Work out the finished part from the listing and answer in its coordinate system (mm). A direction names the side the tool comes from. Round coordinates to 2 decimals unless told otherwise and drop trailing zeros. Answer as CSV lines item,"result". Start each with the question number.
Q1. Each of these flat-tipped pins is pushed along its axis until it touches: pin 1 Ø3 at (x, y) = (-11, 4) entering from +Z; pin 2 Ø0.9 at (y, z) = (4, 151) entering from -X; pin 3 Ø0.5 at (y, z) = (4.5, 140.5) entering from +X; pin 4 Ø3 at (x, y) = (0, 0) entering from -Z. Where does it stop, or does it pass through?
Q2. The mould has two halves that part along Y. Classify faces 4 (the face through (-7, -3.5, 213)), 5 (the face through (-3.5, 2, 213)), 6 (the face through (1.3, 1.9, 0)): +Y half, -Y half, draft (parallel to the pull), parting line (faces both ways), or undercut.
Q3. Straight lines are drawn through the part: L1, parallel to X at y = -0.5, z = 326.5; L2, parallel to Y at x = -11.5, z = 175; L3, parallel to Y at x = 7, z = 354. For each, find the intervals that lie inside material, in ascending order. Write a range as [from, to].
Q4. For faces 1 (the face through (1.3, 1.9, 431.8)), 2 (the face through (11, 2.5, 213)), 3 (the face through (11, 0.5, 213)), determine the directions among +Z, -Z, +X, -X, +Y, -Y from which every point of the face is accessible in a straight line to the end or side of a thin tool.
```python
from build123d import *

# Parameters (mm, degrees)
PAD_DEPTH       = 431.8
FILLET_R        = 1
CHAMFER_SIZE    = 0.5
CHAMFER001_SIZE = 2
FILLET001_R     = 3.5
FILLET002_R     = 1
CHAMFER002_SIZE = 2
FILLET003_R     = 1


with BuildPart() as part:
    # Sketch → Pad (new body)
    with BuildSketch(Plane.XY):
        with BuildLine():
            Line((-13.5, -3.5), (3.75, -3.5))
            Line((3.75, -3.5), (3.75, 0.2))
            Line((3.75, 0.2), (5.75, 0.2))
            Line((5.75, 0.2), (5.75, -3.5))
            Line((5.75, -3.5), (8, -3.5))
            Line((8, -3.5), (8, -1.5))
            Line((8, -1.5), (6.75, -1.5))
            Line((6.75, -1.5), (6.75, 0.5))
            Line((6.75, 0.5), (15.75, 0.5))
            Line((15.75, 0.5), (15.75, -1.5))
            Line((15.75, -1.5), (14.5, -1.5))
            Line((14.5, -1.5), (14.5, -3.5))
            Line((14.5, -3.5), (19.3, -3.5))
            Line((19.3, -3.5), (19.3, -2.5))
            Line((19.3, -2.5), (17.3, -2.5))
            Line((17.3, -2.5), (17.3, -0.7))
            Line((17.3, -0.7), (19.3, -0.7))
            Line((19.3, -0.7), (19.3, 2.5))
            Line((19.3, 2.5), (4.5, 2.5))
            Line((4.5, 2.5), (4.5, 5.25))
            Line((4.5, 5.25), (1, 5.25))
            Line((1, 5.25), (1, 1.732051))
            ThreePointArc((-1, 1.732051), (0, -2), (1, 1.732051))
            Line((-1, 1.732051), (-1, 6.5))
            Line((-1, 6.5), (-16.5, 6.5))
            Line((-16.5, 6.5), (-16.5, 5))
            Line((-16.5, 5), (-13.5, 5))
            Line((-13.5, 5), (-13.5, 3.25))
            Line((-13.5, 3.25), (-11.3, 3.25))
            Line((-11.3, 3.25), (-11.3, 4.15))
            Line((-11.3, 4.15), (-9.5, 4.15))
            Line((-9.5, 4.15), (-9.5, 3.25))
            Line((-9.5, 3.25), (-8.5, 3.25))
            Line((-8.5, 3.25), (-8.5, 5))
            Line((-8.5, 5), (-3.5, 5))
            Line((-3.5, 5), (-3.5, -2))
            Line((-3.5, -2), (-8.5, -2))
            Line((-8.5, -2), (-8.5, -0.25))
            Line((-8.5, -0.25), (-9.5, -0.25))
            Line((-9.5, -0.25), (-9.5, -1.15))
            Line((-9.5, -1.15), (-11.3, -1.15))
            Line((-11.3, -1.15), (-11.3, -0.25))
            Line((-11.3, -0.25), (-13.5, -0.25))
            Line((-13.5, -0.25), (-13.5, -0.45))
            Line((-13.5, -0.45), (-13.3, -0.45))
            Line((-13.3, -0.45), (-13.3, -3.3))
            Line((-13.3, -3.3), (-13.5, -3.3))
            Line((-13.5, -3.3), (-13.5, -3.5))
        make_face()
    extrude(amount=PAD_DEPTH)

    # Fillet
    fillet_edges = [part.edges().sort_by_distance(p)[0] for p in [
        (-1, 6.5, 215.9),
    ]]
    fillet(fillet_edges, radius=FILLET_R)

    # Chamfer
    chamfer_edges = [part.edges().sort_by_distance(p)[0] for p in [
        (4.5, 5.25, 215.9),
    ]]
    chamfer(chamfer_edges, length=CHAMFER_SIZE)

    # Chamfer001
    chamfer001_edges = [part.edges().sort_by_distance(p)[0] for p in [
        (1, 5.25, 215.9),
    ]]
    chamfer(chamfer001_edges, length=CHAMFER001_SIZE)

    # Fillet001
    fillet001_edges = [part.edges().sort_by_distance(p)[0] for p in [
        (3.75, -3.5, 215.9),
    ]]
    fillet(fillet001_edges, radius=FILLET001_R)

    # Fillet002
    fillet002_edges = [part.edges().sort_by_distance(p)[0] for p in [
        (8, -3.5, 215.9),
        (14.5, -3.5, 215.9),
    ]]
    fillet(fillet002_edges, radius=FILLET002_R)

    # Chamfer002
    chamfer002_edges = [part.edges().sort_by_distance(p)[0] for p in [
        (19.3, 2.5, 215.9),
    ]]
    chamfer(chamfer002_edges, length=CHAMFER002_SIZE)

    # Fillet003
    fillet003_edges = [part.edges().sort_by_distance(p)[0] for p in [
        (-16.5, 5, 215.9),
    ]]
    fillet(fillet003_edges, radius=FILLET003_R)


solid = part.part
```
Findings:
1,pin 1,"stops at z = 431.8"
1,pin 2,"stops at x = -13.5"
1,pin 3,"stops at x = 4.5"
1,pin 4,"passes through"
2,face 4,"-Y half"
2,face 5,"undercut"
2,face 6,"draft"
3,L1,"x = [-13.3, -11.3], [-9.5, -8.5], [-3.5, -1.94], [1.94, 3.71], [5.75, 6.75], [15.75, 19.3]"
3,L2,"y = [-3.5, -0.25], [3.25, 6.5]"
3,L3,"y = [-3.5, -1.5], [0.5, 2.5]"
4,face 1,"+Z, +X, -X, +Y, -Y"
4,face 2,"+Z, -Z, +X, +Y"
4,face 3,"+Z, -Z"
